from build123d import *

# Parameters (mm, degrees)
BOSS_EXTRUDE1_DEPTH = 285.75
SKETCH2_R           = 2.4892
CUT_EXTRUDE1_DEPTH  = 25.4
SKETCH3_R           = 2.4892
CUT_EXTRUDE2_DEPTH  = 25.4


with BuildPart() as part:
    # Sketch1 → Boss-Extrude1 (new body)
    with BuildSketch(Plane(origin=(0, 0, 0), x_dir=(1, 0, 0), z_dir=(0, 1, 0))):
        Polygon((6.35, 3.666174209), (0, 7.332348419), (-6.35, 3.666174209), (-6.35, -3.666174209), (0, -7.332348419), (6.35, -3.666174209), align=None)
    extrude(amount=BOSS_EXTRUDE1_DEPTH)

    # Sketch2 → Cut-Extrude1 (cut)
    with BuildSketch(Plane.XZ):
        Circle(SKETCH2_R)
    extrude(amount=-CUT_EXTRUDE1_DEPTH, mode=Mode.SUBTRACT)

    # Sketch3 → Cut-Extrude2 (cut)
    with BuildSketch(Plane(origin=(0, 285.75, 0), x_dir=(1, 0, 0), z_dir=(0, 1, 0))):
        Circle(SKETCH3_R)
    extrude(amount=-CUT_EXTRUDE2_DEPTH, mode=Mode.SUBTRACT)


solid = part.part
Read the model definition and answer for the solid it produces. Units are mm, in the model's axes. A direction names the side the tool comes from. Give positions to 0.01 mm unless a question says otherwise; leave off trailing zeros. Loops run counter-clockwise (first coordinate to the right, second up) from the corner with the lowest first, then second, coordinate; pieces in that order, holes last. Notation, with made-up numbers: (-31.5, 16) - (17.5, 16) arc R17 ccw to (17.5, 35) - close; hole circle Ø11 at (-14, 19). An arc over 180 degrees is marked (long way). Answer as CSV lines item,"result". Start each with the question number.
1) Straight lines are drawn through the part: L1, parallel to X at y = 278.25, z = 0; L2, parallel to Z at x = 0, y = 271.5; L3, parallel to Z at x = -4.75, y = 83.5. For each, find the intervals that lie inside material, in ascending order. Write a range as from..to.
2) Find section B-B (z = 0). Write down the section's boundary in (x, y).
3) Find section A-A (y = 19). Write down the section's boundary in (x, z).
4) Each of these flat-tipped pins is pushed along its axis until it touches: pin 1 Ø2.5 at (x, z) = (-0.5, -0.5) entering from -Y; pin 2 Ø3 at (x, y) = (3.5, 170.5) entering from +Z; pin 3 Ø4 at (x, y) = (3.5, 205.5) entering from -Z. Where does it stop, or does it pass through?
5) Determine the mould class of faces 1 (the face through (6.35, 141, 0)), 2 (the face through (2.374, 273.228, -0.748)), 3 (the face through (-3.131, 140.875, -5.525)) for opening direction Z: released by +Z, released by -Z, zero draft, split by the parting line, or undercut.
6) Which of the six approach directions +Z, -Z, +X, -X, +Y, -Y give full straight-line access (tool end or side, diameter ignored) to faces 4 (the face through (0, 25.4, 0)), 5 (the face through (-3.219, 140.875, 5.474)), 6 (the face through (0, 260.35, 0))?
Findings below:
1,L1,"-6.35..-2.49, 2.49..6.35"
1,L2,"-7.33..-2.49, 2.49..7.33"
1,L3,"-4.59..4.59"
2,outline,"(-6.35, 0) - (-2.49, 0) - (-2.49, 25.4) - (2.49, 25.4) - (2.49, 0) - (6.35, 0) - (6.35, 285.75) - (2.49, 285.75) - (2.49, 260.35) - (-2.49, 260.35) - (-2.49, 285.75) - (-6.35, 285.75) - close"
3,outline,"(-6.35, -3.67) - (0, -7.33) - (6.35, -3.67) - (6.35, 3.67) - (0, 7.33) - (-6.35, 3.67) - close; hole circle Ø4.98 at (0, 0)"
4,pin 1,"y = 25.4"
4,pin 2,"z = 6.18"
4,pin 3,"z = -6.47"
5,face 1,"zero draft"
5,face 2,"undercut"
5,face 3,"released by -Z"
6,face 4,"-Y"
6,face 5,"+Z, -X, +Y, -Y"
6,face 6,"+Y"
